Work out the finished part from the listing and answer in its coordinate system (mm). A direction names the side the tool comes from. Coordinates: 2 decimals unless noted, no trailing zeros. Write each loop counter-clockwise with the first axis right and the second up, starting at its lowest first coordinate (ties: lowest second). Pieces come first, ordered by that corner, then holes. Notation, with made-up numbers: (-16, -17.75) - (18, -17.75) arc R28 ccw to (18, 18.25) - close; hole circle Ø6 at (-36, 73). An arc over 180 degrees is marked (long way). Use CSV: the item, a comma, the result in double quotes. Start each with the question number.
from build123d import *

# Parameters (mm, degrees)
SKETCH1_W           = 31.65
SKETCH1_H           = 59.35
SKETCH1_R           = 4.5
SKETCH1_W_2         = 3.175
SKETCH1_H_2         = 6
BOSS_EXTRUDE1_DEPTH = 5.4
SKETCH2_R           = 4.45936
BOSS_EXTRUDE2_DEPTH = 5.4


with BuildPart() as part:
    # Sketch1 → Boss-Extrude1 (new body)
    with BuildSketch(Plane(origin=(0, 0, 0), x_dir=(1, 0, 0), z_dir=(0, 1, 0))):
        with Locations((-3.498626473, 0.073295681)):
            Rectangle(SKETCH1_W, SKETCH1_H)
        with Locations((-3.498626473, 17.248295681)):
            Circle(SKETCH1_R, mode=Mode.SUBTRACT)
        with Locations((-20.911126473, 3.484009967)):
            Rectangle(SKETCH1_W_2, SKETCH1_H_2)
        with Locations((-20.911126473, -8.558847176)):
            Rectangle(SKETCH1_W_2, SKETCH1_H_2)
        with Locations((-20.911126473, -20.601704319)):
            Rectangle(SKETCH1_W_2, SKETCH1_H_2)
        with Locations((13.913873527, -20.601704319)):
            Rectangle(SKETCH1_W_2, SKETCH1_H_2)
        with Locations((13.913873527, -8.558847176)):
            Rectangle(SKETCH1_W_2, SKETCH1_H_2)
        with Locations((13.913873527, 3.484009967)):
            Rectangle(SKETCH1_W_2, SKETCH1_H_2)
    extrude(amount=BOSS_EXTRUDE1_DEPTH)

    # Sketch2 → Boss-Extrude2 (add)
    with BuildSketch(Plane(origin=(0, 5.4, 0), x_dir=(1, 0, 0), z_dir=(0, 1, 0))):
        Polygon((12.367013527, 6.524649967), (12.367013527, 29.788935681), (-19.364266473, 29.788935681), (-19.364266473, 6.524649967), (-22.539266473, 6.524649967), (-22.539266473, 0.443369967), (-19.364266473, 0.443369967), (-19.364266473, -5.518207176), (-22.539266473, -5.518207176), (-22.539266473, -11.599487176), (-19.364266473, -11.599487176), (-19.364266473, -17.561064319), (-22.539266473, -17.561064319), (-22.539266473, -23.642344319), (-19.364266473, -23.642344319), (-19.364266473, -29.642344319), (12.367013527, -29.642344319), (12.367013527, -23.642344319), (15.542013527, -23.642344319), (15.542013527, -17.561064319), (12.367013527, -17.561064319), (12.367013527, -11.599487176), (15.542013527, -11.599487176), (15.542013527, -5.518207176), (12.367013527, -5.518207176), (12.367013527, 0.443369967), (15.542013527, 0.443369967), (15.542013527, 6.524649967), align=None)
        with Locations((-3.498626473, 17.248295681)):
            Circle(SKETCH2_R, mode=Mode.SUBTRACT)
    extrude(amount=-BOSS_EXTRUDE2_DEPTH)


solid = part.part
Item 1: Each of these flat-tipped pins is pushed along its axis until it touches: pin 1 (2.5 mm diameter, centred on y = 3, z = 27, fed in from -X); pin 2 (1.6 mm diameter, centred on x = -20.5, y = 2, fed in from -Z); pin 3 (1.6 mm diameter, centred on x = -20.5, y = 1.5, fed in from +Z); pin 4 (10 mm diameter, centred on x = 4, z = -6, fed in from -Y). Where does it stop, or does it pass through?
Item 2: Determine the mould class of faces 4 (the face through (-19.364, 3, -18)), 5 (the face through (-21, 3, 17.561)), 6 (the face through (-21, 3, 23.642)) for opening direction Z: +Z half, -Z half, draft (parallel to the pull), parting line (faces both ways), or undercut.
Item 3: Which of the six approach directions +Z, -Z, +X, -X, +Y, -Y give full straight-line access (tool end or side, diameter ignored) to faces 1 (the face through (-19.364, 3, 2)), 2 (the face through (14, 3, 5.518)), 3 (the face through (14, 3, 23.642))?
Item 4: Straight lines are drawn through the part: probe 1 along Z at (x, y) = (-20.5, 3.9); probe 2 along X at (y, z) = (1.25, 14); probe 3 along Z at (x, y) = (-2, 3.9). For each, find the intervals that lie inside material, in ascending order. Write a range as [from, to].
Item 5: A cutting plane is placed at B-B (x = -5.5). Determine the outline of the cut face in (y, z).
Item 6: A cutting plane is placed at C-C (z = -24.5). Determine the outline of the cut face in (x, y), then the cut area to 3 significant figures.
Calculated:
1,pin 1,"stops at x = -19.36"
1,pin 2,"stops at z = -6.52"
1,pin 3,"stops at z = 23.64"
1,pin 4,"stops at y = 0"
2,face 4,"draft"
2,face 5,"undercut"
2,face 6,"+Z half"
3,face 1,"-X, +Y, -Y"
3,face 2,"+X, +Y, -Y"
3,face 3,"+Z, +X, +Y, -Y"
4,probe 1,"z = [-6.52, -0.44], [5.52, 11.6], [17.56, 23.64]"
4,probe 2,"x = [-19.36, 12.37]"
4,probe 3,"z = [-29.79, -21.45], [-13.05, 29.64]"
5,outline,"(0, -29.79) - (5.4, -29.79) - (5.4, -21.23) - (0, -21.23) - close; (0, -13.26) - (5.4, -13.26) - (5.4, 29.64) - (0, 29.64) - close"
6,outline,"(-19.36, 0) - (12.37, 0) - (12.37, 5.4) - (-19.36, 5.4) - close"
6,area,"171 mm²"
